from build123d import *

# Parameters (mm, degrees)
F0_W          = 25.4
F0_H          = 609.6
F1_DEPTH      = 406.4
F2_W          = 342.9
F2_H          = 558.8
F3_DEPTH      = 15.241
F3_DEPTH_BACK = 10.161
F4_W          = 10.16
F4_H          = 69.85
F5_DEPTH      = 406.401
F5_DEPTH_BACK = 406.401


with BuildPart() as f1:
    # F0 (on Right) → F1 (new body, symmetric)
    with BuildSketch(Plane.YZ):
        with Locations((2.54, 234.95)):
            Rectangle(F0_W, F0_H)
    extrude(amount=F1_DEPTH, both=True)

    # F2 (on Front) → F3 (cut, two sides)
    with BuildSketch(Plane.XZ) as f3_sk:
        with Locations((-184.15, 209.55)):
            Rectangle(F2_W, F2_H)
        with Locations((184.15, 209.55)):
            Rectangle(F2_W, F2_H)
    extrude(amount=-F3_DEPTH, mode=Mode.SUBTRACT)
    extrude(f3_sk.sketch, amount=F3_DEPTH_BACK, mode=Mode.SUBTRACT)

    # F4 (on Right) → F5 (cut, two sides)
    with BuildSketch(Plane.YZ) as f5_sk:
        with Locations((-5.08, -34.925)):
            Rectangle(F4_W, F4_H)
    extrude(amount=-F5_DEPTH, mode=Mode.SUBTRACT)
    extrude(f5_sk.sketch, amount=F5_DEPTH_BACK, mode=Mode.SUBTRACT)


solid = f1.part
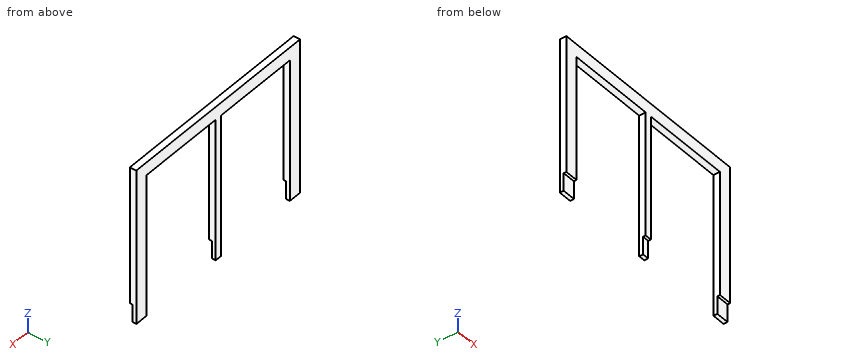
Read the model definition and answer for the solid it produces. Units are mm, in the model's axes. Round coordinates to 2 decimals unless told otherwise and drop trailing zeros. Loops run counter-clockwise (first coordinate to the right, second up) from the corner with the lowest first, then second, coordinate; pieces in that order, holes last. Notation, with made-up numbers: (84.25, 22) - (126.25, 22) arc R27 cw to (126.25, 60) - close; hole circle Ø9 at (58.25, 69). An arc over 180 degrees is marked (long way). One line per question, with ' | ' between items. Start each with the question number.
Q1. Find the intervals of material crossed by L1, parallel to X at y = -5.5, z = 185.5; L2, parallel to Z at x = 258.5, y = -7.5, in increasing order.
Q2. Section B-B on y = -4 is taken. Give the vertices of the cut face in (x, z), plus the area to 3 significant figures.
Q3. Section A-A on z = -14 is taken. Give the vertices of the cut face in (x, y).
Q4. Section D-D on x = 169 is taken. Give the vertices of the cut face in (y, z).
Q5. Flat-ended cylindrical pins translate along their axes: pin 1 (15 mm diameter, centred on x = -393.5, z = -52.5, fed in from -Y); pin 2 (7.5 mm diameter, centred on x = 105, y = 7, fed in from -Z); pin 3 (10 mm diameter, centred on x = 15, y = 1.5, fed in from -Z); pin 4 (5 mm diameter, centred on x = 3, y = -6, fed in from -Z). Find the tip coordinate at first contact, or state that the pin passes through.
Q6. Section C-C on z = 364 is taken. Give the vertices of the cut face in (x, y), plus the area to 3 significant figures.
Established:
1) L1: -406.4 to -355.6, -12.7 to 12.7, 355.6 to 406.4 | L2: 488.95 to 539.75
2) outline: (-406.4, 0) - (-355.6, 0) - (-355.6, 488.95) - (-12.7, 488.95) - (-12.7, 0) - (12.7, 0) - (12.7, 488.95) - (355.6, 488.95) - (355.6, 0) - (406.4, 0) - (406.4, 539.75) - (-406.4, 539.75) - close | area: 103,000 mm²
3) outline: (-406.4, 0) - (-355.6, 0) - (-355.6, 15.24) - (-406.4, 15.24) - close; (-12.7, 0) - (12.7, 0) - (12.7, 15.24) - (-12.7, 15.24) - close; (355.6, 0) - (406.4, 0) - (406.4, 15.24) - (355.6, 15.24) - close
4) outline: (-10.16, 488.95) - (15.24, 488.95) - (15.24, 539.75) - (-10.16, 539.75) - close
5) pin 1: y = 0 | pin 2: z = 488.95 | pin 3: z = -69.85 | pin 4: z = 0
6) outline: (-406.4, -10.16) - (-355.6, -10.16) - (-355.6, 15.24) - (-406.4, 15.24) - close; (-12.7, -10.16) - (12.7, -10.16) - (12.7, 15.24) - (-12.7, 15.24) - close; (355.6, -10.16) - (406.4, -10.16) - (406.4, 15.24) - (355.6, 15.24) - close | area: 3,230 mm²
